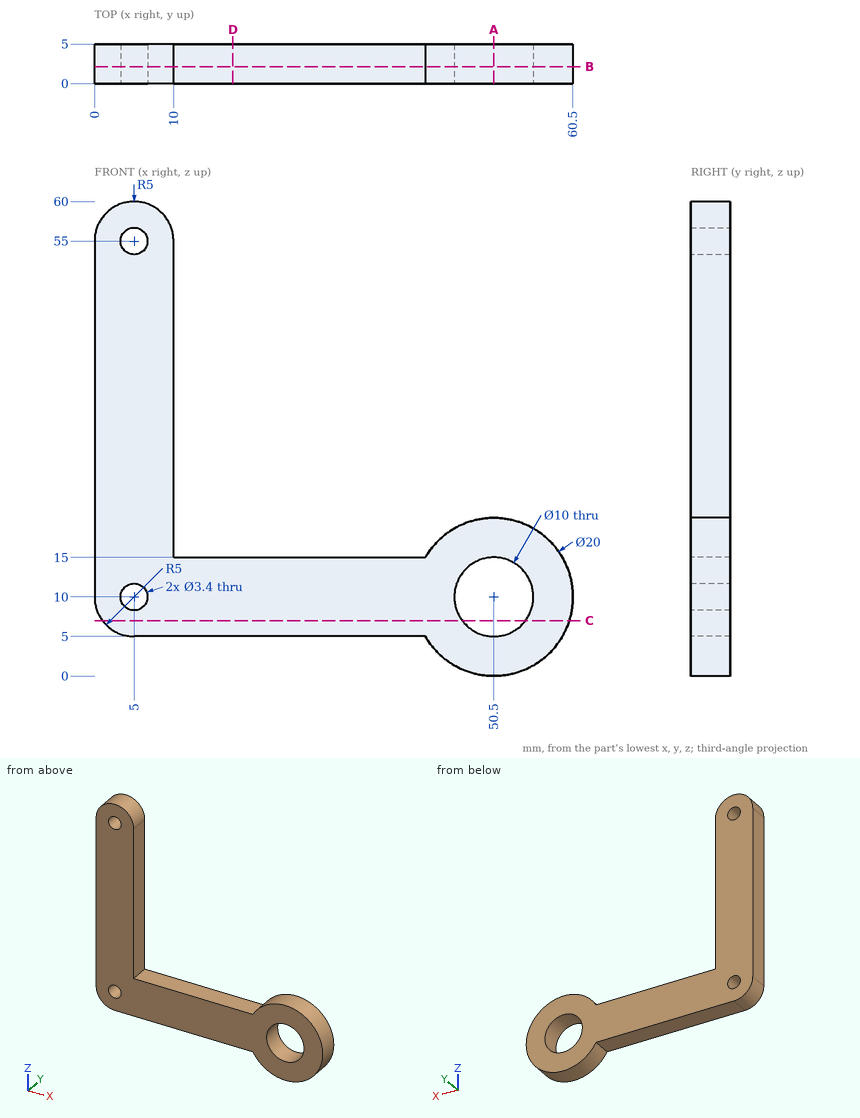
Source: three-view drawing plus pictorial views. Frame: mm from the lowest corner of the part. Give positions to 0.01 mm unless a question says otherwise; leave off trailing zeros. Write each loop counter-clockwise with the first axis right and the second up, starting at its lowest first coordinate (ties: lowest second). Pieces come first, ordered by that corner, then holes. Notation, with made-up numbers: (30, 19.25) - (44, 19.25) arc R30 ccw to (44, 53.25) - close; hole circle Ø5 at (48, 17). An arc over 180 degrees is marked (long way). Write item = value, one per line. Start each with the question number.
1. Ray query, L1, parallel to X at y = 3.85, z = 55; L2, parallel to X at y = 3.75, z = 10; L3, parallel to X at y = 0.8, z = 9. Return the intervals inside material, ascending.
2. Section query A-A, the plane x = 50.5. Output: boundary loops of the cut face in (y, z).
3. First-contact query: pin 1 Ø3 at (y, z) = (3, 26.5) entering from +X; pin 2 Ø2 at (x, z) = (5, 55) entering from +Y; pin 3 Ø1.5 at (x, y) = (48, 1) entering from -Z; pin 4 Ø1.5 at (x, y) = (31, 3.5) entering from -Z. Flat tips, straight axial feed; report the tip coordinate or a pass-through.
4. Section query C-C, the plane z = 7. Output: boundary loops of the cut face in (x, y), then the cut area to 3 significant figures.
5. Section query D-D, the plane x = 17.5. Output: boundary loops of the cut face in (y, z), then the cut area to 3 significant figures.
6. Section query B-B, the plane y = 2.15. Output: boundary loops of the cut face in (x, z).
Check sheet entries:
q1.L1 = 0 to 3.3, 6.7 to 10
q1.L2 = 0 to 3.3, 6.7 to 45.5, 55.5 to 60.5
q1.L3 = 0.1 to 3.63, 6.37 to 45.6, 55.4 to 60.45
q2.outline = (0, 0) - (5, 0) - (5, 5) - (0, 5) - close; (0, 15) - (5, 15) - (5, 20) - (0, 20) - close
q3.pin_1 = 10
q3.pin_2 = through
q3.pin_3 = 0.15
q3.pin_4 = 5
q4.outline = (1, 0) - (46.5, 0) - (46.5, 5) - (1, 5) - close; (54.5, 0) - (60.04, 0) - (60.04, 5) - (54.5, 5) - close
q4.area = 255 mm2
q5.outline = (0, 5) - (5, 5) - (5, 15) - (0, 15) - close
q5.area = 50.0 mm2
q6.outline = (0, 10) arc R5 ccw to (5, 5) - (41.84, 5) arc R10 ccw (long way) to (41.84, 15) - (10, 15) - (10, 55) arc R5 ccw to (0, 55) - close; hole circle Ø3.4 at (5, 10); hole circle Ø3.4 at (5, 55); hole circle Ø10 at (50.5, 10)
